Geometry check sheet. Reference: the model listing, model coordinates, mm. A direction names the side the tool comes from. Round coordinates to 2 decimals unless told otherwise and drop trailing zeros. Write each loop counter-clockwise with the first axis right and the second up, starting at its lowest first coordinate (ties: lowest second). Pieces come first, ordered by that corner, then holes.
from build123d import *

# Parameters (mm, degrees)
SKETCH1_R           = 1.1
BOSS_EXTRUDE1_DEPTH = 5
BOSS_EXTRUDE2_DEPTH = 5
BOSS_EXTRUDE3_DEPTH = 9
SKETCH5_R           = 1
CUT_EXTRUDE1_DEPTH  = 16
SKETCH6_R           = 1.9
CUT_EXTRUDE2_DEPTH  = 1
FILLET1_R           = 0.5
SKETCH7_W           = 5
SKETCH7_H           = 16
BOSS_EXTRUDE4_DEPTH = 9
FILLET2_R           = 7


with BuildPart() as part:
    # Sketch1 → Boss-Extrude1 (new body)
    with BuildSketch(Plane.XY):
        with BuildLine():
            ThreePointArc((0, 4.5), (-4.5, 0), (0, -4.5))
            Line((0, -4.5), (7, -4.5))
            ThreePointArc((7, -4.5), (42.961642557, 14.118622766), (80.916317371, 0))
            Line((80.916317371, 0), (90, 0))
            Line((90, 0), (90, 4.5))
            Line((90, 4.5), (85, 4.5))
            ThreePointArc((85, 4.5), (46, 20.654328933), (7, 4.5))
            Line((7, 4.5), (0, 4.5))
        make_face()
        Circle(SKETCH1_R, mode=Mode.SUBTRACT)
    extrude(amount=BOSS_EXTRUDE1_DEPTH)

    # Sketch3 → Boss-Extrude2 (add)
    with BuildSketch(Plane.XY.offset(5)):
        Polygon((90, 0), (90, -4.5), (85, -4.5), (80.916317371, 0), align=None)
    extrude(amount=-BOSS_EXTRUDE2_DEPTH)

    # Sketch4 → Boss-Extrude3 (add)
    with BuildSketch(Plane(origin=(0, 4.5, 0), x_dir=(1, 0, 0), z_dir=(0, 1, 0))):
        Polygon((90.5, 2), (100, 2), (100, 5.5), (90, 5.5), (90, 0), (90, -5), (90, -10.5), (100, -10.5), (100, -7), (90.5, -7), align=None)
    extrude(amount=-BOSS_EXTRUDE3_DEPTH)

    # Sketch5 → Cut-Extrude1 (cut)
    with BuildSketch(Plane(origin=(0, 0, -5.5), x_dir=(-1, 0, 0), z_dir=(0, 0, -1))):
        with Locations((-96, 0)):
            Circle(SKETCH5_R)
    extrude(amount=-CUT_EXTRUDE1_DEPTH, mode=Mode.SUBTRACT)

    # Sketch6 → Cut-Extrude2 (cut)
    with BuildSketch(Plane(origin=(0, 0, -5.5), x_dir=(-1, 0, 0), z_dir=(0, 0, -1))):
        with Locations((-96, 0)):
            Circle(SKETCH6_R)
    extrude(amount=-CUT_EXTRUDE2_DEPTH, mode=Mode.SUBTRACT)

    # Fillet1
    fillet1_edges = [part.edges().sort_by_distance(p)[0] for p in [
        (97, 0, 7),
    ]]
    fillet(fillet1_edges, radius=FILLET1_R)

    # Sketch7 → Boss-Extrude4 (add)
    with BuildSketch(Plane.XZ.offset(4.5)):
        with Locations((87.5, 2.5)):
            Rectangle(SKETCH7_W, SKETCH7_H)
    extrude(amount=-BOSS_EXTRUDE4_DEPTH)

    # Fillet2
    # the kernel refuses this fillet: 7 mm, written as the material it adds along each edge
    with BuildSketch(Plane(origin=(85, 21.593492914, 0), x_dir=(0, 0, -1), z_dir=(0, -1, 0))) as fillet2_piece_1_section:
        with BuildLine():
            CenterArc((7, -6.837397166), FILLET2_R, 102.373625116, 77.626374884)
            Line((0, -6.837397166), (0, 0))
            Line((0, 0), (5.5, 0))
        make_face()
    fillet2_piece_1 = extrude(amount=43.186985828, mode=Mode.PRIVATE)
    fillet2_piece_1 = fillet2_piece_1 & Plane(origin=(46, -34.5, 0), x_dir=(0.7071067811865476, 0.7071067811865476, 0), z_dir=(0, 0, -1)) * Cylinder(55.154328933, 114, mode=Mode.PRIVATE)
    fillet2_piece_1 = split(fillet2_piece_1, bisect_by=Plane(origin=(72.014490495, 9.809337449, 0), z_dir=(0.7405316990978602, 0.6720214301874877, 0)), keep=Keep.TOP, mode=Mode.PRIVATE)
    add(fillet2_piece_1)
    with BuildSketch(Plane(origin=(85, 4.5, 0), x_dir=(0, 0, -1), z_dir=(0, -1, 0))) as fillet2_piece_2_section:
        with BuildLine():
            CenterArc((7, -6.837397166), FILLET2_R, 102.373625116, 77.626374884)
            Line((0, -6.837397166), (0, 0))
            Line((0, 0), (5.5, 0))
        make_face()
    fillet2_piece_2 = extrude(amount=26.093492914, mode=Mode.PRIVATE)
    fillet2_piece_2 = fillet2_piece_2 - Plane(origin=(46, -35.788975694, 0), x_dir=(-0.7799999999999994, 0.6257795138864816, 0), z_dir=(0, 0, -1)) * Cylinder(50, 80, mode=Mode.PRIVATE)
    add(fillet2_piece_2)
    with BuildSketch(Plane(origin=(85, 21.593492914, 5), x_dir=(-1, 0, 0), z_dir=(0, -1, 0))) as fillet2_piece_3_section:
        with BuildLine():
            CenterArc((6.837397166, -7), FILLET2_R, 90, 77.626374884)
            Line((0, -5.5), (0, 0))
            Line((0, 0), (6.837397166, 0))
        make_face()
    fillet2_piece_3 = extrude(amount=43.186985828, mode=Mode.PRIVATE)
    fillet2_piece_3 = fillet2_piece_3 & Plane(origin=(46, -34.5, 5), x_dir=(0.7071067811865476, 0.7071067811865476, 0), z_dir=(0, 0, -1)) * Cylinder(55.154328933, 114, mode=Mode.PRIVATE)
    fillet2_piece_3 = split(fillet2_piece_3, bisect_by=Plane(origin=(72.014490495, 9.809337449, 5), z_dir=(0.7405316990978602, 0.6720214301874877, 0)), keep=Keep.TOP, mode=Mode.PRIVATE)
    add(fillet2_piece_3)
    with BuildSketch(Plane(origin=(85, 4.5, 5), x_dir=(-1, 0, 0), z_dir=(0, -1, 0))) as fillet2_piece_4_section:
        with BuildLine():
            CenterArc((6.837397166, -7), FILLET2_R, 90, 77.626374884)
            Line((0, -5.5), (0, 0))
            Line((0, 0), (6.837397166, 0))
        make_face()
    fillet2_piece_4 = extrude(amount=26.093492914, mode=Mode.PRIVATE)
    fillet2_piece_4 = fillet2_piece_4 - Plane(origin=(46, -35.788975694, 5), x_dir=(-0.7799999999999994, 0.6257795138864816, 0), z_dir=(0, 0, -1)) * Cylinder(50, 80, mode=Mode.PRIVATE)
    add(fillet2_piece_4)


solid = part.part
1. Section check A-A (x = 96). Record the cut outline in (y, z).
2. Release check for a two-part mould opening along Y. For faces 6 (the face through (34, 14, 0)), 7 (the face through (97.9, 0.08, -5.01)), 8 (the face through (89, 4.5, 3)), 9 (the face through (95, -1, -4.5)) record: +Y half, -Y half, draft (parallel to the pull), parting line (faces both ways), or undercut.
3. Section check B-B (z = 3). Record the cut outline in (x, y), plus the area to 3 significant figures.
4. Scan lines: line 1 along Y through (x, z) = (96, -5.05); line 2 along Y through (x, z) = (96, 9.85); line 3 along Y through (x, z) = (5.5, 0.25). Record each from-to range of solid material in increasing order.
5. Access from +Z, -Z, +X, -X, +Y, -Y to the whole of each face (thin tool, end or side, straight path). Record for faces 1 (the face through (34, 14, 5)), 2 (the face through (92, 0, 10.5)), 3 (the face through (100, 0, 9)), 4 (the face through (90.5, 0, 3)), 5 (the face through (4, 4.5, 2)).
6. Section check D-D (x = 2.5). Record the cut outline in (y, z), plus the area to 3 significant figures.
7. Depth check by flat-ended pin: pin 1 Ø6 at (x, y) = (96, 0) entering from -Z; pin 2 Ø6 at (x, z) = (32.5, -0.5) entering from -Y; pin 3 Ø2.5 at (x, y) = (96, 0) entering from -Z; pin 4 Ø2.5 at (y, z) = (0.5, 2) entering from +X. Enter the tip coordinate at first touch or a pass-through.
8. Section check C-C (y = 6.75). Record the cut outline in (x, z), plus the area to 3 significant figures.
Results below:
1. outline: (-4.5, -5.5) - (-1.9, -5.5) - (-1.9, -4.5) - (-1, -4.5) - (-1, -2) - (-4.5, -2) - close; (-4.5, 7) - (-1.5, 7) arc R0.5 ccw to (-1, 7.5) - (-1, 10.5) - (-4.5, 10.5) - close; (1, -4.5) - (1.9, -4.5) - (1.9, -5.5) - (4.5, -5.5) - (4.5, -2) - (1, -2) - close; (1, 7.5) arc R0.5 ccw to (1.5, 7) - (4.5, 7) - (4.5, 10.5) - (1, 10.5) - close
2. face 6: draft
2. face 7: undercut
2. face 8: +Y half
2. face 9: undercut
3. outline: (0, -4.5) - (7, -4.5) arc R50 cw to (80.92, 0) - (85, -4.5) - (90.5, -4.5) - (90.5, 4.5) - (85, 4.5) arc R55.15 ccw to (7, 4.5) - (0, 4.5) arc R4.5 ccw to start; hole circle Ø2.2 at (0, 0)
3. area: 695 mm2
4. line 1: y = -4.5 to -1.9, 1.9 to 4.5
4. line 2: y = -4.5 to -1, 1 to 4.5
4. line 3: y = -4.5 to 4.5
5. face 1: +Z, -X, +Y, -Y
5. face 2: +Z, +X, -X, +Y, -Y
5. face 3: +Z, -Z, +X, +Y, -Y
5. face 4: +X, +Y, -Y
5. face 5: +Z, -Z, -X, +Y
6. outline: (-4.5, 0) - (4.5, 0) - (4.5, 5) - (-4.5, 5) - close
6. area: 45.0 mm2
7. pin 1: stops at z = -5.5
7. pin 2: stops at y = 11.42
7. pin 3: stops at z = -4.5
7. pin 4: stops at x = 90.5
8. outline: (9.39, 0) - (19.72, 0) - (19.72, 5) - (9.39, 5) - close; (72.28, 0) - (78.16, 0) arc R7 cw to (82.61, -1.6) - (82.61, 6.6) arc R7 cw to (78.16, 5) - (72.28, 5) - close
8. area: 108 mm2
